```python
from build123d import *

# Parameters (mm, degrees)
F2_SIZE2 = 0.8
F2_SIZE  = 0.8
F3_R     = 0.8
F5_DEPTH = 6.4


with BuildPart() as f1:
    # F0 (on Top) → F1 (revolve)
    with BuildSketch(Plane.XY):
        Polygon((90.3, 0), (0, 0), (0, -8), (1.5, -8), (1.5, -5), (90.3, -5), align=None)
    revolve(axis=Axis((45.15, 0, 0), (1, 0, 0)))

    # F2
    f2_edges = [f1.edges().sort_by_distance(p)[0] for p in [
        (90.3, 5, 0),
    ]]
    chamfer(f2_edges, length=F2_SIZE, length2=F2_SIZE2)

    # F3
    f3_edges = [f1.edges().sort_by_distance(p)[0] for p in [
        (0, 8, 0),
    ]]
    fillet(f3_edges, radius=F3_R)

    # F4 (on face) → F5 (cut)
    with BuildSketch(Plane(origin=(0, 0, 0), x_dir=(0, -1, 0), z_dir=(-1, 0, 0))):
        Polygon((2.502813, -1.445), (2.502813, 1.445), (0, 2.89), (-2.502813, 1.445), (-2.502813, -1.445), (0, -2.89), align=None)
    extrude(amount=-F5_DEPTH, mode=Mode.SUBTRACT)


solid = f1.part
```
Geometry: final body of the model. Coordinates: model frame, mm. A direction names the side the tool comes from. Round coordinates to 2 decimals unless told otherwise and drop trailing zeros. Loops run counter-clockwise (first coordinate to the right, second up) from the corner with the lowest first, then second, coordinate; pieces in that order, holes last. Notation, with made-up numbers: (69, -11) -> (103, -11) arc R27 ccw to (103, 18) -> close; hole circle Ø8 at (72, 86.5). An arc over 180 degrees is marked (long way). Use one line per item in the form item = value.
Item 1: Material intervals for probe 1 along Y at (x, z) = (49, 0); probe 2 along X at (y, z) = (-1.75, 5.25); probe 3 along X at (y, z) = (-1, 0.5), sorted ascending.
Evaluation:
probe_1 = -5 to 5
probe_2 = 0 to 1.5
probe_3 = 6.4 to 90.3
Item 2: Cut plane A-A on z = 0. Output: boundary loops of the cut face in (x, y).
Evaluation:
outline = (0, -7.2) arc R0.8 ccw to (0.8, -8) -> (1.5, -8) -> (1.5, -5) -> (89.5, -5) -> (90.3, -4.2) -> (90.3, 4.2) -> (89.5, 5) -> (1.5, 5) -> (1.5, 8) -> (0.8, 8) arc R0.8 ccw to (0, 7.2) -> (0, 2.5) -> (6.4, 2.5) -> (6.4, -2.5) -> (0, -2.5) -> close
Item 3: Draft query along Z for faces 4 (the cylindrical face through (46.12, 1.08, 4.88)), 5 (the flat face through (3, 2.503, 0)), 6 (the flat face through (0, -0.1, 3.1)). Return one class per face: released by +Z, released by -Z, zero draft, split by the parting line, or undercut.
Evaluation:
face_4 = split by the parting line
face_5 = undercut
face_6 = zero draft
Item 4: Cut plane B-B on x = 69. Output: boundary loops of the cut face in (y, z), then the cut area to 3 significant figures.
Evaluation:
outline = circle Ø10 at (0, 0)
area = 78.5 mm2
Item 5: Contact query for flat-ended pins moving along their axis: pin 1 Ø0.9 at (x, z) = (3, 0) entering from +Y; pin 2 Ø3 at (x, y) = (78, -3) entering from +Z; pin 3 Ø3 at (x, z) = (4.5, 0.5) entering from -Y. Output: stop coordinate, or through.
Evaluation:
pin_1 = 5
pin_2 = 4.77
pin_3 = -5
Item 6: Access query for faces 1 (the flat face through (1.5, 0.1, 5.2)), 2 (the flat face through (3, -2.503, 0)), 3 (the flat face through (90.3, 0, 0)). Directions: +Z, -Z, +X, -X, +Y, -Y. A direction counts if a zero-diameter tool reaches every point of the face in a straight line with its end or side. Return the directions, or none.
Evaluation:
face_1 = +X
face_2 = -X
face_3 = +Z, -Z, +X, +Y, -Y
